from build123d import *

# Parameters (mm, degrees)
BOSS_EXTRUDE1_DEPTH   = 3.175
F_3_0MM_DOWEL_HOLE1_D = 3
FILLET1_R             = 1


with BuildPart() as part:
    # Sketch1 → Boss-Extrude1 (new body)
    with BuildSketch(Plane.XY):
        Polygon((0, 2), (0, -2), (5, -2), (5, -5), (36.1, -5), (36.1, -2), (41.1, -2), (41.1, 2), (36.1, 2), (36.1, 5), (5, 5), (5, 2), align=None)
    extrude(amount=BOSS_EXTRUDE1_DEPTH)

    # Ø3.0mm Dowel Hole1 (through all)
    with Locations(Plane.XY.offset(3.175)):
        with Locations((10, 0), (31.1, 0)):
            Hole(F_3_0MM_DOWEL_HOLE1_D / 2)

    # Fillet1
    fillet1_edges = [part.edges().sort_by_distance(p)[0] for p in [
        (0, -2, 1.5875),
        (0, 2, 1.5875),
        (5, 5, 1.5875),
        (36.1, 5, 1.5875),
        (41.1, 2, 1.5875),
        (41.1, -2, 1.5875),
        (36.1, -5, 1.5875),
        (5, -5, 1.5875),
    ]]
    fillet(fillet1_edges, radius=FILLET1_R)


solid = part.part
Could you check a few things on this model? Use its own coordinates, in mm. A direction names the side the tool comes from. Round coordinates to 2 decimals unless told otherwise and drop trailing zeros. Write each loop counter-clockwise with the first axis right and the second up, starting at its lowest first coordinate (ties: lowest second). Pieces come first, ordered by that corner, then holes. Notation, with made-up numbers: (-16, -18.75) - (8, -18.75) arc R28 ccw to (8, 18.25) - close; hole circle Ø1 at (36.5, 23.25). An arc over 180 degrees is marked (long way). Use a Markdown table: item, result.
Q1. For faces 1 (the flat face through (36.1, 3, 2)), 2 (the flat face through (3, -2, 2)), 3 (the flat face through (5, 3, 2)), which set-ups out of +Z, -Z, +X, -X, +Y, -Y let a thin tool reach every point of the face, with its end or its side?
Output values:
| item | result |
|---|---|
| face 1 | +Z, -Z, +X, +Y |
| face 2 | +Z, -Z, -X, -Y |
| face 3 | +Z, -Z, -X, +Y |
Q2. I want a section at D-D (x = 38.5). List the corners of the cut face in (y, z) for me (3 decimals).
Output values:
| item | result |
|---|---|
| outline | (-2, 0) - (2, 0) - (2, 3.175) - (-2, 3.175) - close |
Q3. I want a section at C-C (z = 2.8). List the corners of the cut face in (x, y) for me.
Output values:
| item | result |
|---|---|
| outline | (0, -1) arc R1 ccw to (1, -2) - (5, -2) - (5, -4) arc R1 ccw to (6, -5) - (35.1, -5) arc R1 ccw to (36.1, -4) - (36.1, -2) - (40.1, -2) arc R1 ccw to (41.1, -1) - (41.1, 1) arc R1 ccw to (40.1, 2) - (36.1, 2) - (36.1, 4) arc R1 ccw to (35.1, 5) - (6, 5) arc R1 ccw to (5, 4) - (5, 2) - (1, 2) arc R1 ccw to (0, 1) - close; hole circle Ø3 at (10, 0); hole circle Ø3 at (31.1, 0) |
Q4. I want a section at A-A (x = 31.1). List the corners of the cut face in (y, z) for me (3 decimals), plus the area to 3 significant figures.
Output values:
| item | result |
|---|---|
| outline | (-5, 0) - (-1.5, 0) - (-1.5, 3.175) - (-5, 3.175) - close; (1.5, 0) - (5, 0) - (5, 3.175) - (1.5, 3.175) - close |
| area | 22.2 mm2 |
Q5. I want a section at B-B (y = 0). List the corners of the cut face in (x, z) for me (3 decimals), plus the area to 3 significant figures.
Output values:
| item | result |
|---|---|
| outline | (0, 0) - (8.5, 0) - (8.5, 3.175) - (0, 3.175) - close; (11.5, 0) - (29.6, 0) - (29.6, 3.175) - (11.5, 3.175) - close; (32.6, 0) - (41.1, 0) - (41.1, 3.175) - (32.6, 3.175) - close |
| area | 111 mm2 |
Q6. For pin 1 (1 mm diameter, centred on y = -3.5, z = 1, fed in from +X); pin 2 (1.6 mm diameter, centred on x = 39, z = 1.5, fed in from -Y); pin 3 (1 mm diameter, centred on y = 3, z = 2, fed in from -X), each with a flat end and sliding along its axis, tell me the tip position at first contact or that it passes through.
Output values:
| item | result |
|---|---|
| pin 1 | x = 36.1 |
| pin 2 | y = -2 |
| pin 3 | x = 5 |
Q7. Please list where these lines run through material, in increasing order: L1, parallel to Y at x = 31.1, z = 1.4; L2, parallel to X at y = -1, z = 2.55; L3, parallel to X at y = 3, z = 1.7.
Output values:
| item | result |
|---|---|
| L1 | -5 to -1.5, 1.5 to 5 |
| L2 | 0 to 8.88, 11.12 to 29.98, 32.22 to 41.1 |
| L3 | 5 to 36.1 |
Q8. Thinking about a two-plate mould opening in X: for faces 4 (the cylindrical face through (40.799, -1.715, 1.61)), 5 (the cylindrical face through (29.67, 0.45, 1.57)), 6 (the flat face through (20, 0, 0)), 7 (the cylindrical face through (5.285, -4.699, 1.61)), which applies, released by +X, released by -X, zero draft, split by the parting line, or undercut?
Output values:
| item | result |
|---|---|
| face 4 | released by +X |
| face 5 | undercut |
| face 6 | zero draft |
| face 7 | released by -X |
